Source: CAD feature listing. Evaluate the final solid. Frame: model axes, mm. A direction names the side the tool comes from. Round coordinates to 2 decimals unless told otherwise and drop trailing zeros. Write each loop counter-clockwise with the first axis right and the second up, starting at its lowest first coordinate (ties: lowest second). Pieces come first, ordered by that corner, then holes.
from build123d import *

# Parameters (mm, degrees)
SKETCH_1_W          = 50
SKETCH_1_H          = 80
EXTRUDE_1_DEPTH     = 5
SKETCH_2_W          = 50
SKETCH_2_H          = 80
EXTRUDE_2_DEPTH     = 5
EXTRUDE_3_DEPTH     = 5
SKETCH_4_R          = 4
CUT_EXTRUDE_1_DEPTH = 94.674969976
SKETCH_5_R          = 4
CUT_EXTRUDE_2_DEPTH = 119.215904175
FILLET_1_R          = 25


with BuildPart() as part:
    # Sketch 1 → Extrude 1 (new body)
    with BuildSketch(Plane.XY):
        Rectangle(SKETCH_1_W, SKETCH_1_H)
    extrude(amount=EXTRUDE_1_DEPTH)



with BuildPart() as body_2:
    # Sketch 2 → Extrude 2 (new body)
    with BuildSketch(Plane.XY.offset(65)):
        Rectangle(SKETCH_2_W, SKETCH_2_H)
    extrude(amount=EXTRUDE_2_DEPTH)


with BuildPart() as part_1:
    add(part.part)

    add(body_2.part)  # Extrude 3 merges body 2
    # Sketch 3 → Extrude 3 (add)
    with BuildSketch(Plane(origin=(0, 40, 0), x_dir=(1, 0, 0), z_dir=(0, 1, 0))):
        with BuildLine():
            Line((-25, 0), (25, 0))
            ThreePointArc((25, 0), (43.011626335, -35), (25, -70))
            Line((25, -70), (-25, -70))
            ThreePointArc((-25, -70), (-43.011626335, -35), (-25, 0))
        make_face()
    extrude(amount=EXTRUDE_3_DEPTH)

    # Sketch 4 → Cut-Extrude 1 (cut, through all)
    with BuildSketch(Plane.XY.offset(70)):
        with Locations((0, -20)):
            Circle(SKETCH_4_R)
    extrude(amount=-CUT_EXTRUDE_1_DEPTH, mode=Mode.SUBTRACT)

    # Sketch 5 → Cut-Extrude 2 (cut, through all)
    with BuildSketch(Plane(origin=(0, 45, 0), x_dir=(1, 0, 0), z_dir=(0, 1, 0))):
        with Locations(Location((0, -35, 0), (0, 0, 180))):
            Circle(SKETCH_5_R)
    extrude(amount=-CUT_EXTRUDE_2_DEPTH, mode=Mode.SUBTRACT)

    # Fillet 1
    fillet_1_edges = [part_1.edges().sort_by_distance(p)[0] for p in [
        (-25, -40, 2.5),
        (25, -40, 2.5),
        (25, -40, 67.5),
        (-25, -40, 67.5),
    ]]
    fillet(fillet_1_edges, radius=FILLET_1_R - 0.0001)  # a hair under: the kernel refuses the full size


solid = part_1.part
1) Contact query for flat-ended pins moving along their axis: P1, Ø15, axis at x = 5, y = 16.5, coming from the -Z side; P2, Ø8, axis at x = -28.5, z = 25, coming from the -Y side; P3, Ø4, axis at y = 25.5, z = 66.5, coming from the -X side; P4, Ø4, axis at y = 5.5, z = 3.5, coming from the +X side. Output: stop coordinate, or through.
Taken from the geometry:
P1: stops at z = 0
P2: stops at y = 40
P3: stops at x = -25
P4: stops at x = 25
2) Pull-direction query (X, two-part tool) for faces 1 (the face through (1, 45, 42)), 2 (the face through (0.521, 42.535, 38.966)), 3 (the face through (-43, 42, 36)); classes: released by +X, released by -X, zero draft, split by the parting line, or undercut.
Taken from the geometry:
face 1: zero draft
face 2: undercut
face 3: released by -X
3) Section query C-C on y = -20. Return the cut outline in (x, z), then the cut area to 3 significant figures.
Taken from the geometry:
outline: (-24.49, 0) - (-4, 0) - (-4, 5) - (-24.49, 5) - close; (-24.49, 65) - (-4, 65) - (-4, 70) - (-24.49, 70) - close; (4, 0) - (24.49, 0) - (24.49, 5) - (4, 5) - close; (4, 65) - (24.49, 65) - (24.49, 70) - (4, 70) - close
area: 410 mm2
4) Section query B-B on y = 26.5. Return the cut outline in (x, z).
Taken from the geometry:
outline: (-25, 0) - (25, 0) - (25, 5) - (-25, 5) - close; (-25, 65) - (25, 65) - (25, 70) - (-25, 70) - close
5) Section query A-A on z = 35. Return the cut outline in (x, y), then the cut area to 3 significant figures.
Taken from the geometry:
outline: (-43.01, 40) - (-4, 40) - (-4, 45) - (-43.01, 45) - close; (4, 40) - (43.01, 40) - (43.01, 45) - (4, 45) - close
area: 390 mm2
6) Section query D-D on x = -13. Return the cut outline in (y, z).
Taken from the geometry:
outline: (-36.35, 0) - (45, 0) - (45, 70) - (-36.35, 70) - (-36.35, 65) - (40, 65) - (40, 5) - (-36.35, 5) - close
7) Reachability of faces 4 (the face through (-25, 12, 67)), 5 (the face through (0, 1, 5)), 6 (the face through (25, 12, 2)), 7 (the face through (-0.521, -16.034, 2.535)) from +Z, -Z, +X, -X, +Y, -Y: full face, straight path, thin tool, end or side. Return the list, or none.
Taken from the geometry:
face 4: +Z, -Z, -X, -Y
face 5: +X, -X, -Y
face 6: +Z, -Z, +X, -Y
face 7: +Z, -Z
8) Material intervals for line 1 (Z direction, x = -20.5, y = -12); line 2 (Y direction, x = 0, z = 66.6); line 3 (Y direction, x = 8, z = 54.5), sorted ascending.
Taken from the geometry:
line 1: z = 0 to 5, 65 to 70
line 2: y = -40 to -24, -16 to 45
line 3: y = 40 to 45
